from build123d import *

# Parameters (mm, degrees)
SKETCH_1_R          = 17.29
SKETCH_1_R_2        = 1.1
SKETCH_1_R_3        = 2.5
EXTRUDE_1_DEPTH     = 4
SKETCH_2_W          = 4
SKETCH_2_H          = 4.8
SKETCH_2_H_2        = 3.4
SKETCH_2_W_2        = 4.4
SKETCH_2_H_3        = 4
SKETCH_2_W_3        = 18
SKETCH_2_H_4        = 12
CUT_EXTRUDE_1_DEPTH = 1.6
SKETCH_3_R          = 17.29
SKETCH_3_R_2        = 2.5
SKETCH_3_R_3        = 1.1
EXTRUDE_2_DEPTH     = 1
SKETCH_4_W          = 10
SKETCH_4_H          = 15
CUT_EXTRUDE_2_DEPTH = 1.4


with BuildPart() as part:
    # 草图1 → 凸台-拉伸1 (new body)
    with BuildSketch(Plane(origin=(0, 0, 0), x_dir=(1, 0, 0), z_dir=(0, 1, 0))):
        with Locations(Location((0, 0, 0), (0, 0, 270))):
            Circle(SKETCH_1_R)
        with Locations(Location((-13.72, 0, 0), (0, 0, 270))):
            Circle(SKETCH_1_R_2, mode=Mode.SUBTRACT)
        with Locations(Location((13.72, 0, 0), (0, 0, 270))):
            Circle(SKETCH_1_R_2, mode=Mode.SUBTRACT)
        with Locations(Location((-4.85, 9.64, 0), (0, 0, 270))):
            Circle(SKETCH_1_R_3, mode=Mode.SUBTRACT)
        with BuildLine():
            Line((-12.309220648, 6.98), (-7.690779352, 6.98))
            ThreePointArc((-7.690779352, 6.98), (-7.35, 5.68), (-7.690779352, 4.38))
            Line((-7.690779352, 4.38), (-12.309220648, 4.38))
            ThreePointArc((-12.309220648, 4.38), (-12.65, 5.68), (-12.309220648, 6.98))
        make_face(mode=Mode.SUBTRACT)
        with BuildLine():
            Line((12.309220648, 6.98), (7.690779352, 6.98))
            ThreePointArc((7.690779352, 6.98), (7.35, 5.68), (7.690779352, 4.38))
            Line((7.690779352, 4.38), (12.309220648, 4.38))
            ThreePointArc((12.309220648, 4.38), (12.65, 5.68), (12.309220648, 6.98))
        make_face(mode=Mode.SUBTRACT)
    extrude(amount=EXTRUDE_1_DEPTH)

    # 草图2 → 切除-拉伸1 (cut)
    with BuildSketch(Plane.XZ):
        with Locations((-7.22, 0.9)):
            Rectangle(SKETCH_2_W, SKETCH_2_H)
        with Locations((8, -1.1)):
            Rectangle(SKETCH_2_W, SKETCH_2_H_2)
        with Locations((-14.996048965, 3.8)):
            Rectangle(SKETCH_2_W_2, SKETCH_2_H_3)
        with Locations((0, 11.29)):
            Rectangle(SKETCH_2_W_3, SKETCH_2_H_4)
    extrude(amount=-CUT_EXTRUDE_1_DEPTH, mode=Mode.SUBTRACT)

    # 草图3 → 凸台-拉伸2 (add)
    with BuildSketch(Plane(origin=(0, 4, 0), x_dir=(1, 0, 0), z_dir=(0, 1, 0))):
        with Locations(Location((0, 0, 0), (0, 0, 185.97568604))):
            Circle(SKETCH_3_R)
        with Locations(Location((-4.85, 9.64, 0), (0, 0, 270))):
            Circle(SKETCH_3_R_2, mode=Mode.SUBTRACT)
        with Locations(Location((-13.72, 0, 0), (0, 0, 270))):
            Circle(SKETCH_3_R_3, mode=Mode.SUBTRACT)
        with Locations(Location((13.72, 0, 0), (0, 0, 270))):
            Circle(SKETCH_3_R_3, mode=Mode.SUBTRACT)
    extrude(amount=EXTRUDE_2_DEPTH)

    # 草图4 → 切除-拉伸2 (cut)
    with BuildSketch(Plane(origin=(0, 5, 0), x_dir=(1, 0, 0), z_dir=(0, 1, 0))):
        with Locations((-10.82, 8.9)):
            Rectangle(SKETCH_4_W, SKETCH_4_H)
    extrude(amount=-CUT_EXTRUDE_2_DEPTH, mode=Mode.SUBTRACT)


solid = part.part
Geometry: final body of the model. Coordinates: model frame, mm. A direction names the side the tool comes from. Coordinates: 2 decimals unless noted, no trailing zeros. Loops run counter-clockwise (first coordinate to the right, second up) from the corner with the lowest first, then second, coordinate; pieces in that order, holes last. Notation, with made-up numbers: (60, 27) - (64, 27) arc R21 cw to (64, 41) - close; hole circle Ø9 at (88, 72). An arc over 180 degrees is marked (long way). One line per question, with ' | ' between items. Start each with the question number.
(1) Ray query, L1, parallel to X at y = 1.1, z = 0; L2, parallel to X at y = 1.8, z = 0; L3, parallel to Z at x = -4.85, y = 1.15. Return the intervals inside material, ascending. Write a range as from..to.
(2) Draft query along X for faces 6 (the flat face through (9, 1, 10)), 7 (the flat face through (0, 0, -5)), 8 (the cylindrical face through (-8.057, 4.132, 15.298)). Return one class per face: +X half, -X half, draft (parallel to the pull), parting line (faces both ways), or undercut.
(3) Cut plane D-D on z = -8. Output: boundary loops of the cut face in (x, y), and give its area (3 significant figures).
(4) Cut plane C-C on x = 13.72. Output: boundary loops of the cut face in (y, z), and give its area (3 significant figures).
(5) Reachability of faces 1 (the flat face through (-15.82, 4, -4)), 2 (the flat face through (-5.82, 4, -14)), 3 (the flat face through (8, 1, 0.6)), 4 (the flat face through (0, 1.6, 11)), 5 (the flat face through (-10, 2, -6.98)) from +Z, -Z, +X, -X, +Y, -Y: full face, straight path, thin tool, end or side. Return the list, or none.
(6) First-contact query: pin 1 (1.3 mm diameter, centred on x = 3, y = 1, fed in from +Z); pin 2 (10 mm diameter, centred on x = 11.5, z = 0, fed in from -Y); pin 3 (3 mm diameter, centred on x = -10.5, y = 2, fed in from +Z); pin 4 (3 mm diameter, centred on x = -12, z = -9, fed in from +Y). Flat tips, straight axial feed; report the tip coordinate or a pass-through.
(7) Cut plane B-B on z = 0. Output: boundary loops of the cut face in (x, y), and give its area (3 significant figures).
(8) Cut plane A-A on y = 0.55. Output: boundary loops of the cut face in (x, z).
Here are the results:
1) L1: -17.29..-14.82, -12.62..-9.22, -5.22..6, 10..12.62, 14.82..17.29 | L2: -17.29..-14.82, -12.62..12.62, 14.82..17.29 | L3: -16.6..-12.14, -7.14..5.29
2) face 6: undercut | face 7: draft | face 8: parting line
3) outline: (-15.33, 0) - (-6.74, 0) - (-6.74, 3.6) - (-15.33, 3.6) - close; (-2.96, 0) - (15.33, 0) - (15.33, 5) - (-2.96, 5) - close | area: 122 mm²
4) outline: (0, -10.52) - (5, -10.52) - (5, -1.1) - (0, -1.1) - close; (0, 1.1) - (5, 1.1) - (5, 10.52) - (0, 10.52) - close | area: 94.2 mm²
5) face 1: -Z, +Y | face 2: -Z, -X, +Y | face 3: -Y | face 4: +Z, -Y | face 5: +Y, -Y
6) pin 1: z = 17.07 | pin 2: y = 0 | pin 3: z = 14.76 | pin 4: y = 3.6
7) outline: (-17.29, 0) - (-14.82, 0) - (-14.82, 5) - (-17.29, 5) - close; (-12.62, 0) - (-9.22, 0) - (-9.22, 1.6) - (-5.22, 1.6) - (-5.22, 0) - (6, 0) - (6, 1.6) - (10, 1.6) - (10, 0) - (12.62, 0) - (12.62, 5) - (-12.62, 5) - close; (14.82, 0) - (17.29, 0) - (17.29, 5) - (14.82, 5) - close | area: 138 mm²
8) outline: (-17.2, 1.8) arc R17.29 ccw (long way) to (9, 14.76) - (9, 5.29) - (-9, 5.29) - (-9, 14.76) arc R17.29 ccw to (-16.29, 5.8) - (-12.8, 5.8) - (-12.8, 1.8) - close; hole circle Ø2.2 at (-13.72, 0); hole (-12.31, -6.98) - (-7.69, -6.98) arc R2.65 ccw to (-7.69, -4.38) - (-12.31, -4.38) arc R2.65 ccw to start; hole (-9.22, -1.5) - (-5.22, -1.5) - (-5.22, 3.3) - (-9.22, 3.3) - close; hole circle Ø5 at (-4.85, -9.64); hole (6, -2.8) - (10, -2.8) - (10, 0.6) - (6, 0.6) - close; hole (7.69, -6.98) - (12.31, -6.98) arc R2.65 ccw to (12.31, -4.38) - (7.69, -4.38) arc R2.65 ccw to start; hole circle Ø2.2 at (13.72, 0)
